Geometry check sheet. Reference: drawing and pictorial views, mm from the part's lowest x, y, z. A direction names the side the tool comes from. Give positions to 0.01 mm unless a question says otherwise; leave off trailing zeros. Order: outer loops, then holes, each group sorted by start corner. A loop starts at its lowest first (then second) coordinate and runs counter-clockwise, first axis right, second up.
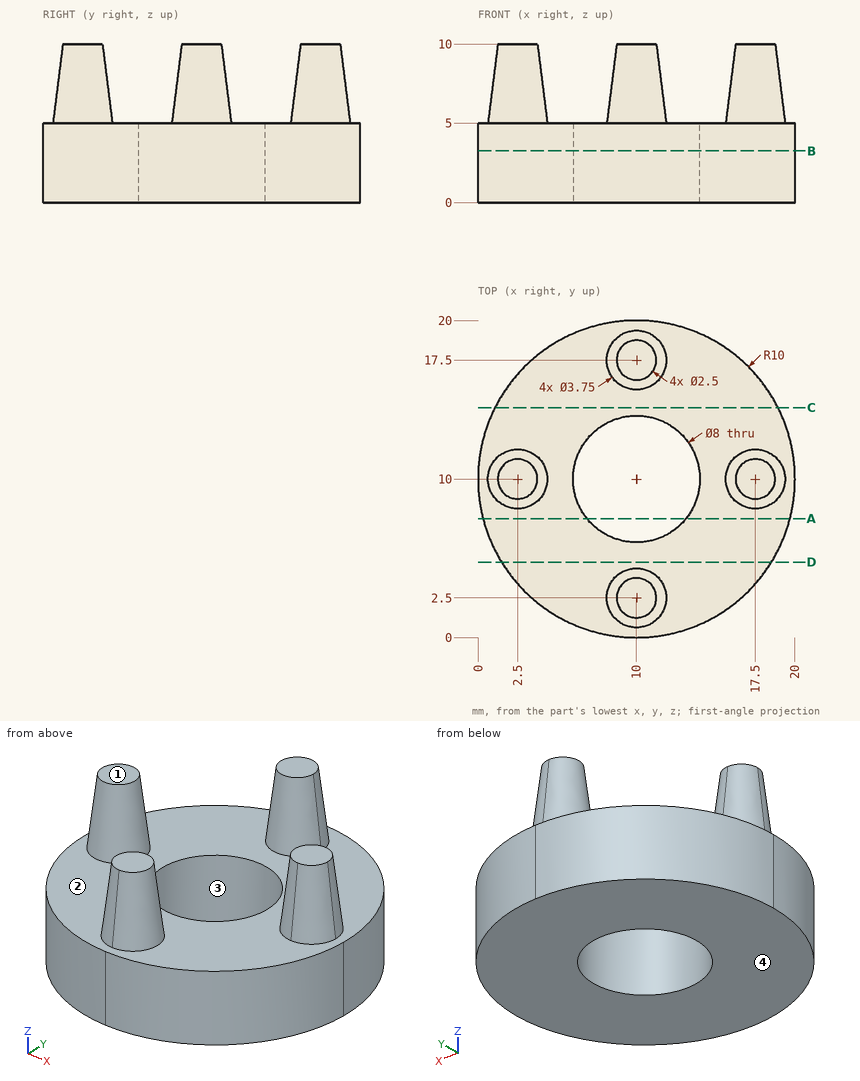
(1) Material ranges on L1, parallel to Z at x = 12.5, y = 3.5; L2, parallel to X at y = 8.75, z = 8.5; L3, parallel to Y at x = 15.75, z = 3.75, recorded low to high.
Response values:
L1: z = 0 to 5
L2: x = 1.79 to 3.21, 16.79 to 18.21
L3: y = 1.82 to 18.18
(2) Cross-section at A-A on y = 7.5. Enter the section's corners in (x, z), then the cut area to 3 significant figures.
Response values:
outline: (0.32, 0) - (6.88, 0) - (6.88, 5) - (0.32, 5) - close; (13.12, 0) - (19.68, 0) - (19.68, 5) - (13.12, 5) - close
area: 65.6 mm2
(3) Cross-section at B-B on z = 3.25. Enter the section's corners in (x, y), then the cut area to 3 significant figures.
Response values:
outline: circle Ø20 at (10, 10); hole circle Ø8 at (10, 10)
area: 264 mm2
(4) Cross-section at C-C on y = 14.5. Enter the section's corners in (x, z).
Response values:
outline: (1.07, 0) - (18.93, 0) - (18.93, 5) - (1.07, 5) - close
(5) Gauge pin test, flat ends, axial feed: pin 1 Ø6 at (x, z) = (17, 3) entering from +Y; pin 2 Ø6 at (y, z) = (2.5, 2) entering from -X; pin 3 Ø3 at (x, y) = (12.5, 7) entering from +Z. Record the tip position at first contact, or that the pin passes through.
Response values:
pin 1: stops at y = 19.17
pin 2: stops at x = 1.07
pin 3: stops at z = 5
(6) Release check for a two-part mould opening along Y. For the marked faces 3 and 4 record: released by +Y, released by -Y, zero draft, split by the parting line, or undercut.
Response values:
face 3: undercut
face 4: zero draft
(7) Set-up check for the marked faces 1 and 2: record each of +Z, -Z, +X, -X, +Y, -Y from which the full face is reachable in a straight line by a thin tool's end or side.
Response values:
face 1: +Z, +X, -X, +Y, -Y
face 2: +Z
(8) Cross-section at D-D on y = 4.75. Enter the section's corners in (x, z), then the cut area to 3 significant figures.
Response values:
outline: (1.49, 0) - (18.51, 0) - (18.51, 5) - (1.49, 5) - close
area: 85.1 mm2
